from build123d import *

# Parameters (mm, degrees)
F1_DEPTH = 190.5
F2_W     = 12
F2_H     = 12
F3_DEPTH = 2
F4_SIZE  = 0.8
F5_DEPTH = 1
F6_R     = 0.4


with BuildPart() as f1:
    # F0 (on Right) → F1 (new body, symmetric)
    with BuildSketch(Plane.YZ):
        with BuildLine():
            Line((-164.7787988186, -76.2), (111.1195152746, -76.2))
            Line((111.1195152746, -76.2), (111.1195152746, 0))
            Line((111.1195152746, 0), (85.7195152746, 0))
            Line((85.7195152746, 0), (85.7195152746, -6.3575065629))
            Line((85.7195152746, -6.3575065629), (68.9104866383, -25.4))
            Line((68.9104866383, -25.4), (-158.9419270625, -43.8726167807))
            ThreePointArc((-158.9419270625, -43.8726167807), (-163.0968211166, -45.8969616661), (-164.7787988186, -50.2018504946))
            Line((-164.7787988186, -50.2018504946), (-164.7787988186, -76.2))
        make_face()
    extrude(amount=F1_DEPTH, both=True)

    # F2 (on face) → F3 (join)
    with BuildSketch(Plane(origin=(0, 2.4957770492, -30.7844216917), x_dir=(1, 0, 0), z_dir=(0, -0.0808075975, 0.9967297187))):
        with Locations((-138.6103741825, -100.1955993752)):
            Rectangle(F2_W, F2_H)
    extrude(amount=F3_DEPTH)

    # F4
    f4_edges = [f1.edges().sort_by_distance(p)[0] for p in [
        (-138.610374, -91.553391, -36.402682),
        (-144.610374, -97.53377, -36.887528),
        (-138.610374, -103.514148, -37.372374),
        (-132.610374, -97.53377, -36.887528),
    ]]
    chamfer(f4_edges, length=F4_SIZE)

    # F5 (add): a face of the model
    f5_faces = [f1.faces().sort_by_distance(p)[0] for p in [
        (-138.6103741825, -97.5337697285, -36.8875279164),
    ]]
    extrude(f5_faces, amount=F5_DEPTH)

    # F6
    f6_edges = [f1.edges().sort_by_distance(p)[0] for p in [
        (-138.610374, -92.431583, -35.470599),
        (-133.410374, -97.614577, -35.890798),
        (-143.810374, -97.614577, -35.890798),
        (-138.610374, -102.797572, -36.310998),
    ]]
    fillet(f6_edges, radius=F6_R)


solid = f1.part
Geometry: final body of the model. Coordinates: model frame, mm. Coordinates: 2 decimals unless noted, no trailing zeros. Loops run counter-clockwise (first coordinate to the right, second up) from the corner with the lowest first, then second, coordinate; pieces in that order, holes last. Notation, with made-up numbers: M -31.75,23 L 1.25,23 A32 ccw 1.25,62 Z; hole C 10,26 d7. An arc over 180 degrees is marked long. One line per item, written item: value. Start each with the question number.
1) Draft query along X for faces 1 (the flat face through (2.667, -43.421, -34.507)), 2 (the flat face through (190.5, 2, -54)), 3 (the flat face through (-190.5, 2, -54)). Return one class per face: released by +X, released by -X, zero draft, split by the parting line, or undercut.
2) Material intervals for L1, parallel to Y at x = 75.5, z = -3; L2, parallel to Z at x = -28, y = -90.5; L3, parallel to Z at x = -97, y = -104, sorted ascending. Write a range as from..to.
3) Cut plane A-A (x = -107). Return loops of the section in (y, z).
4) Pin query (flat end, axial travel): P1, Ø6, axis at x = 98.5, y = -77, coming from the +Z side; P2, Ø1.1, axis at y = -99, z = -38.5, coming from the -X side; P3, Ø10, axis at x = 152, y = -58, coming from the +Z side; P4, Ø1.2, axis at y = -98.5, z = -36.5, coming from the +X side. Return the tip coordinate at first contact, or that it passes through.
5) Cut plane B-B (y = 31.5). Return loops of the section in (x, z).
6) Cut plane C-C (z = -30). Return loops of the section in (x, y).
Evaluation:
1. face 1: zero draft
1. face 2: released by +X
1. face 3: released by -X
2. L1: 85.72..111.12
2. L2: -76.2..-38.32
2. L3: -76.2..-39.42
3. outline: M -164.78,-76.2 L 111.12,-76.2 L 111.12,0 L 85.72,0 L 85.72,-6.36 L 68.91,-25.4 L -158.94,-43.87 A6.35 ccw -164.78,-50.2 Z
4. P1: z = -36.99
4. P2: x = -190.5
4. P3: z = -35.28
4. P4: x = -133.27
5. outline: M -190.5,-76.2 L 190.5,-76.2 L 190.5,-28.43 L -190.5,-28.43 Z
6. outline: M -190.5,12.17 L 190.5,12.17 L 190.5,111.12 L -190.5,111.12 Z
